Here's the drawing with two shaded views (mm, measured from the low corner). I have some questions. Round coordinates to 2 decimals unless told otherwise and drop trailing zeros. Loops run counter-clockwise (first coordinate to the right, second up) from the corner with the lowest first, then second, coordinate; pieces in that order, holes last.
(1) I want a section at C-C on z = 54.5. Write out the boundary of the cut face in (x, y), plus the area to 3 significant figures.
(2) If I drill on line 1 along X through (y, z) = (15.75, 43); line 2 along X through (y, z) = (12.75, 39.5); line 3 along Y through (x, z) = (17.75, 78.5) (1 decimal), over which ranges is the centre line in solid material (lowest first)?
(3) Thinking about a two-plate mould opening in Z: for the marked faces 1, 2, 3 and 4, which applies, released by +Z, released by -Z, zero draft, split by the parting line, or undercut?
(4) I want a section at B-B on x = 15. Write out the boundary of the cut face in (y, z).
(5) I want a section at A-A on z = 84. Write out the boundary of the cut face in (x, y).
(6) Will these pins go through, and if not, where does the flat tip stop? pin 1 Ø5 at (y, z) = (4.5, 21) entering from -X; pin 2 Ø4 at (x, z) = (17, 43) entering from +Y; pin 3 Ø1 at (x, y) = (16.5, 1) entering from +Z; pin 4 Ø16.5 at (x, z) = (15, 53) entering from -Y.
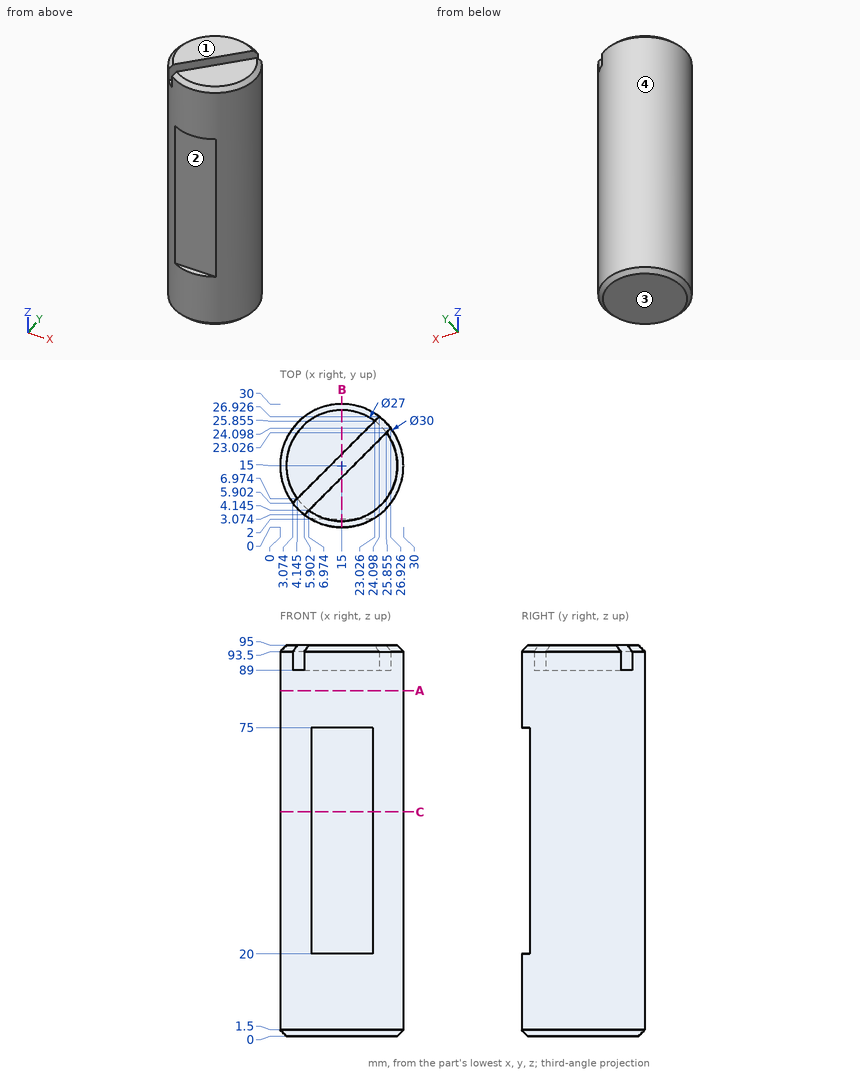
Filled sheet:
1. outline: (7.52, 2) - (22.48, 2) arc R15 ccw (long way) to start
1. area: 687 mm2
2. line 1: x = 0.02 to 29.98
2. line 2: x = 0.17 to 29.83
2. line 3: y = 0.3 to 29.7
3. face 1: released by +Z
3. face 2: undercut
3. face 3: released by -Z
3. face 4: zero draft
4. outline: (0, 1.5) - (1.5, 0) - (28.5, 0) - (30, 1.5) - (30, 93.5) - (28.5, 95) - (17.83, 95) - (17.83, 89) - (12.17, 89) - (12.17, 95) - (1.5, 95) - (0, 93.5) - (0, 75) - (2, 75) - (2, 20) - (0, 20) - close
5. outline: circle Ø30 at (15, 15)
6. pin 1: stops at x = 2.31
6. pin 2: stops at y = 30
6. pin 3: stops at z = 94.92
6. pin 4: stops at y = 2
